Build history of the part. All positions in model axes, mm. A direction names the side the tool comes from. Give positions to 0.01 mm unless a question says otherwise; leave off trailing zeros. Write each loop counter-clockwise with the first axis right and the second up, starting at its lowest first coordinate (ties: lowest second). Pieces come first, ordered by that corner, then holes.
from build123d import *

# Parameters (mm, degrees)
F0_R     = 18.5
F1_DEPTH = 142
F0_R_2   = 22.5
F2_DEPTH = 50
F3_R     = 5
F4_DEPTH = 25
F5_SIZE  = 2


with BuildPart() as f1:
    # F0 (on Right) → F1 (new body)
    with BuildSketch(Plane.YZ):
        Circle(F0_R)
    extrude(amount=F1_DEPTH)

    # F0 (on Right) → F2 (join)
    with BuildSketch(Plane.YZ):
        Circle(F0_R_2)
        Circle(F0_R, mode=Mode.SUBTRACT)
    extrude(amount=F2_DEPTH)

    # F3 (on Front) → F4 (cut, symmetric)
    with BuildSketch(Plane.XZ):
        with Locations((90, 0)):
            Circle(F3_R)
    extrude(amount=F4_DEPTH, both=True, mode=Mode.SUBTRACT)

    # F5
    f5_edges = [f1.edges().sort_by_distance(p)[0] for p in [
        (0, -22.5, 0),
    ]]
    chamfer(f5_edges, length=F5_SIZE)


solid = f1.part
(1) Saw through at D-D, the plane x = 40.5. List the corners of the cut face in (y, z), plus the area to 3 significant figures.
(2) Saw through at B-B, the plane y = 0. List the corners of the cut face in (x, z), plus the area to 3 significant figures.
(3) 3-axis set-ups, long thin cutter, end or side, ignore diameter. For faces 5 (the face through (95.356, 17.089, -7.086)), 6 (the face through (142, 0, 0)): which of +Z, -Z, +X, -X, +Y, -Y reach the whole face in a straight line?
(4) Saw through at A-A, the plane z = 0. List the corners of the cut face in (x, y).
(5) Probe line 1 (X direction, y = -3, z = 0); line 2 (Z direction, x = 90, y = 1); line 3 (X direction, y = -10, z = 17). List the from-to ranges inside material, lowest first.
(6) Saw through at C-C, the plane x = 90. List the corners of the cut face in (y, z).
(7) Drop flat-ended pins along their axis: pin 1 (2 mm diameter, centred on x = 118.5, y = 5.5, fed in from +Z); pin 2 (5 mm diameter, centred on x = 64.5, y = -3, fed in from -Z); pin 3 (1.5 mm diameter, centred on x = 79.5, y = 17.5, fed in from -Z). Give the stop position or say it passes through.
(8) Mould opens along X. For faces 1 (the face through (50, -5, -18)), 2 (the face through (94.619, -0.259, -1.915)), 3 (the face through (25.664, 10.382, -19.961)), 4 (the face through (0, 0, 0)) say: +X half, -X half, draft (parallel to the pull), parting line (faces both ways), or undercut.
Computed values:
1. outline: circle Ø45 at (0, 0)
1. area: 1,590 mm2
2. outline: (0, -20.5) - (2, -22.5) - (50, -22.5) - (50, -18.5) - (142, -18.5) - (142, 18.5) - (50, 18.5) - (50, 22.5) - (2, 22.5) - (0, 20.5) - close; hole circle Ø10 at (90, 0)
2. area: 5,570 mm2
3. face 5: +X
3. face 6: +Z, -Z, +X, +Y, -Y
4. outline: (0, -20.5) - (2, -22.5) - (50, -22.5) - (50, -18.5) - (85, -18.5) - (85, 18.5) - (50, 18.5) - (50, 22.5) - (2, 22.5) - (0, 20.5) - close; (95, -18.5) - (142, -18.5) - (142, 18.5) - (95, 18.5) - close
5. line 1: x = 0 to 85, 95 to 142
5. line 2: z = -18.47 to -5, 5 to 18.47
5. line 3: x = 0 to 50
6. outline: (-17.81, -5) arc R18.5 ccw to (17.81, -5) - close; (-17.81, 5) - (17.81, 5) arc R18.5 ccw to start
7. pin 1: stops at z = 17.94
7. pin 2: stops at z = -18.49
7. pin 3: stops at z = -7.85
8. face 1: +X half
8. face 2: undercut
8. face 3: draft
8. face 4: -X half
